For this review, use the dimensioned drawing (mm, ordinates from the lowest corner) and the shaded views. A direction names the side the tool comes from. Coordinates: 2 decimals unless noted, no trailing zeros. Loops run counter-clockwise (first coordinate to the right, second up) from the corner with the lowest first, then second, coordinate; pieces in that order, holes last. Notation, with made-up numbers: M 9,85.5 L 28,85.5 A12 ccw 28,104.5 Z; hole C -9.5,71 d1. An arc over 180 degrees is marked long. Write item = value, one per line. Start each with the question number.
Q1. Mouldability with a two-part tool opening along X and no side actions: class the marked faces 3, 4 and 5 as released by +X, released by -X, zero draft, split by the parting line, or undercut.
Q2. We need section C-C on x = 21. Give the boundary of the cut face in (y, z).
Q3. We need section A-A on y = 12.7. Give the boundary of the cut face in (x, z).
Q4. Clearance check with flat-ended pins moving along their axes: pin 1 Ø3.5 at (x, y) = (12.7, 22.225) entering from -Z; pin 2 Ø4 at (x, y) = (20.95, 7.94) entering from +Z; pin 3 Ø4.5 at (x, y) = (12.7, 12.7) entering from +Z; pin 4 Ø8 at (y, z) = (4.5, 16) entering from +X. State where each tip first meets the part, or that it passes through.
Q5. We need section D-D on z = 10.5. Give the boundary of the cut face in (x, y), and give its area (3 significant figures).
Q6. We need section B-B on x = 12.7. Count the separate pieces of the cut face and the enclosed holes in it, and give its area (3 significant figures).
Q7. Wall thickness on probe 1 along Y at (x, z) = (12.7, 1.6) (1 decimal); probe 2 along Y at (x, z) = (12.7, 9.25): over which ranges is each line inside the solid? List them lowest first.
Q8. For the marked faces 1 and 2, list the 3-axis set-ups (+Z, -Z, +X, -X, +Y, -Y) from which the entire face can be reached by the end or side of a thin tool; tool diameter is ignored.
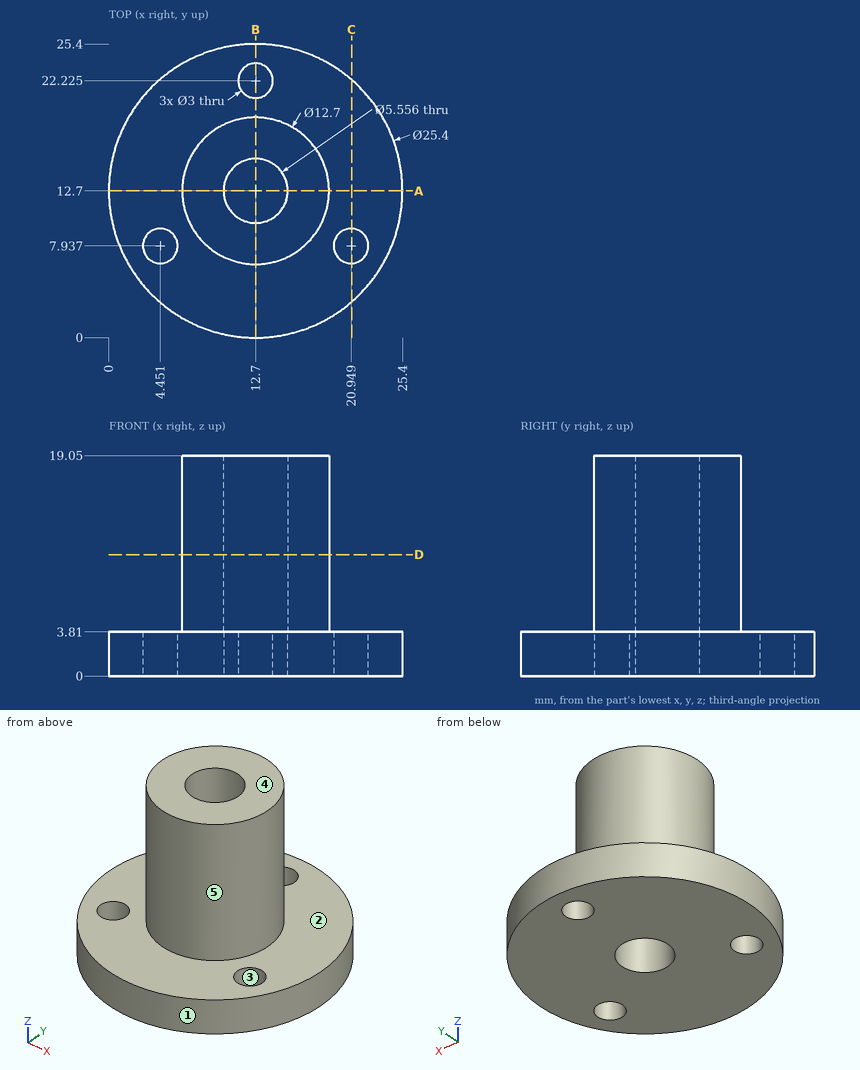
Returned:
q1.face_3 = undercut
q1.face_4 = zero draft
q1.face_5 = split by the parting line
q2.outline = M 3.09,0 L 6.44,0 L 6.44,3.81 L 3.09,3.81 Z; M 9.44,0 L 22.31,0 L 22.31,3.81 L 9.44,3.81 Z
q3.outline = M 0,0 L 9.92,0 L 9.92,19.05 L 6.35,19.05 L 6.35,3.81 L 0,3.81 Z; M 15.48,0 L 25.4,0 L 25.4,3.81 L 19.05,3.81 L 19.05,19.05 L 15.48,19.05 Z
q4.pin_1 = 0
q4.pin_2 = 3.81
q4.pin_3 = through
q4.pin_4 = 17.46
q5.outline = C 12.7,12.7 d12.7; hole C 12.7,12.7 d5.56
q5.area = 102 mm^2
q6.separate_pieces = 3
q6.enclosed_holes = 0
q6.area = 173 mm^2
q7.probe_1 = 0 to 9.9, 15.5 to 20.7, 23.7 to 25.4
q7.probe_2 = 6.35 to 9.92, 15.48 to 19.05
q8.face_1 = +Z, -Z
q8.face_2 = +Z
